```python
from build123d import *

# Parameters (mm, degrees)
F0_W     = 22
F0_H     = 15
F1_DEPTH = 1.5
F2_R     = 1
F3_DEPTH = 1.501
F4_SIZE  = 0.5


with BuildPart() as f1:
    # F0 (on Top) → F1 (new body)
    with BuildSketch(Plane.XY):
        with Locations((11, 7.5)):
            Rectangle(F0_W, F0_H)
    extrude(amount=F1_DEPTH)

    # F2 (on face) → F3 (cut, through all)
    with BuildSketch(Plane.XY.offset(1.5)):
        with Locations((4, 7.5)):
            Circle(F2_R)
        with Locations((8, 7.5)):
            Circle(F2_R)
        with Locations((14, 7.5)):
            Circle(F2_R)
        with Locations((18, 7.5)):
            Circle(F2_R)
    extrude(amount=-F3_DEPTH, mode=Mode.SUBTRACT)

    # F4
    f4_edges = [f1.edges().sort_by_distance(p)[0] for p in [
        (0, 7.5, 1.5),
        (11, 15, 1.5),
        (11, 0, 1.5),
        (22, 7.5, 1.5),
        (3, 7.5, 1.5),
        (7, 7.5, 1.5),
        (13, 7.5, 1.5),
        (17, 7.5, 1.5),
        (0, 7.5, 0),
        (11, 15, 0),
        (11, 0, 0),
        (22, 7.5, 0),
        (3, 7.5, 0),
        (7, 7.5, 0),
        (13, 7.5, 0),
        (17, 7.5, 0),
    ]]
    chamfer(f4_edges, length=F4_SIZE)


solid = f1.part
```
Verification items for the finished model (mm, model axes). Give positions to 0.01 mm unless a question says otherwise; leave off trailing zeros. Loops run counter-clockwise (first coordinate to the right, second up) from the corner with the lowest first, then second, coordinate; pieces in that order, holes last. Notation, with made-up numbers: M -26,53.5 L 8,53.5 A19 cw 8,85.5 Z; hole C 35.25,84 d9. An arc over 180 degrees is marked long. One line per question, with ' | ' between items.
Item 1: Depth check by flat-ended pin: P1, Ø1.6, axis at x = 18, y = 7.5, coming from the +Z side (1 decimal). Enter the tip coordinate at first touch or a pass-through.
Completed:
P1: passes through
Item 2: Section check B-B, the plane y = 3. Record the cut outline in (x, z).
Completed:
outline: M 0,0.5 L 0.5,0 L 21.5,0 L 22,0.5 L 22,1 L 21.5,1.5 L 0.5,1.5 L 0,1 Z
Item 3: Section check C-C, the plane x = 5.75. Record the cut outline in (y, z), plus the area to 3 significant figures.
Completed:
outline: M 0,0.5 L 0.5,0 L 14.5,0 L 15,0.5 L 15,1 L 14.5,1.5 L 0.5,1.5 L 0,1 Z | area: 22.0 mm^2
Item 4: Section check D-D, the plane y = 7.5. State how many separate pieces and enclosed holes the cut face has, plus the area to 3 significant figures.
Completed:
separate pieces: 5 | enclosed holes: 0 | area: 18.5 mm^2
Item 5: Thickness scan on line 1 (X direction, y = 8, z = 0.8); line 2 (Y direction, x = 8, z = 0.6); line 3 (X direction, y = 7.75, z = 0.2). Record the ranges inside material, lowest first. Write a range as [from, to].
Completed:
line 1: x = [0, 3.13], [4.87, 7.13], [8.87, 13.13], [14.87, 17.13], [18.87, 22] | line 2: y = [0, 6.5], [8.5, 15] | line 3: x = [0.3, 2.72], [5.28, 6.72], [9.28, 12.72], [15.28, 16.72], [19.28, 21.7]
Item 6: Section check A-A, the plane x = 18. Record the cut outline in (y, z), plus the area to 3 significant figures.
Completed:
outline: M 0,0.5 L 0.5,0 L 6,0 L 6.5,0.5 L 6.5,1 L 6,1.5 L 0.5,1.5 L 0,1 Z; M 8.5,0.5 L 9,0 L 14.5,0 L 15,0.5 L 15,1 L 14.5,1.5 L 9,1.5 L 8.5,1 Z | area: 18.5 mm^2
Item 7: Draft check along X on faces 1 (the face through (11, 8, 1.5)), 2 (the face through (14.954, 7.8, 0.754)). Enter one of: +X half, -X half, draft (parallel to the pull), parting line (faces both ways), or undercut.
Completed:
face 1: draft | face 2: undercut
